Input: part model. Units: mm. Frame: model coordinates. A direction names the side the tool comes from. Give positions to 0.01 mm unless a question says otherwise; leave off trailing zeros. Order: outer loops, then holes, each group sorted by start corner. A loop starts at its lowest first (then second) coordinate and runs counter-clockwise, first axis right, second up.
```python
from build123d import *

# Parameters (mm, degrees)
PAD001_DEPTH    = 7.5
POCKET_DEPTH    = 17.001
CHAMFER002_SIZE = 0.5
CHAMFER003_SIZE = 0.5
FILLET002_R     = 0.5
FILLET003_R     = 0.5


with BuildPart() as part:
    # Sketch002 → Pad001 (new body, symmetric)
    with BuildSketch(Plane.XY):
        with BuildLine():
            ThreePointArc((-6.5, 3.741657), (0, -7.5), (6.5, 3.741657))
            ThreePointArc((8.233333, 4.739433), (6.867779, 5.107212), (6.5, 3.741657))
            ThreePointArc((7.690476, -5.577327), (9.486876, -0.49919), (8.233333, 4.739433))
            ThreePointArc((7.690476, -5.577327), (7.54881, -5.855807), (7.5, -6.164414))
            Line((7.5, -11.5), (7.5, -6.164414))
            Line((-7.5, -11.5), (7.5, -11.5))
            Line((-7.5, -6.164414), (-7.5, -11.5))
            ThreePointArc((-7.5, -6.164414), (-7.54881, -5.855807), (-7.690476, -5.577327))
            ThreePointArc((-8.233333, 4.739433), (-9.486876, -0.49919), (-7.690476, -5.577327))
            ThreePointArc((-6.5, 3.741657), (-6.867779, 5.107212), (-8.233333, 4.739433))
        make_face()
    extrude(amount=PAD001_DEPTH, both=True)

    # Sketch003 (on Face6 of Pad001) → Pocket (cut, through all)
    with BuildSketch(Plane.YZ.offset(7.5)):
        Polygon((-11.5, -3.237009), (-11.5, 3.237009), (-8.1, 5.2), (-8.1, -5.2), align=None)
    extrude(amount=-POCKET_DEPTH, mode=Mode.SUBTRACT)

    # Chamfer002
    chamfer002_edges = [part.edges().sort_by_distance(p)[0] for p in [
        (7.5, -11.5, 5.368505),
        (7.5, -9.8, 4.218505),
        (7.5, -8.1, 0),
        (7.5, -9.8, -4.218505),
        (7.5, -11.5, -5.368505),
    ]]
    chamfer(chamfer002_edges, length=CHAMFER002_SIZE)

    # Chamfer003
    chamfer003_edges = [part.edges().sort_by_distance(p)[0] for p in [
        (-7.5, -11.5, -5.368505),
        (-7.5, -9.8, -4.218505),
        (-7.5, -8.1, 0),
        (-7.5, -9.8, 4.218505),
        (-7.5, -11.5, 5.368505),
    ]]
    chamfer(chamfer003_edges, length=CHAMFER003_SIZE)

    # Fillet002
    fillet002_edges = [part.edges().sort_by_distance(p)[0] for p in [
        (6.867779, 5.107212, -7.5),
    ]]
    fillet(fillet002_edges, radius=FILLET002_R)

    # Fillet003
    fillet003_edges = [part.edges().sort_by_distance(p)[0] for p in [
        (6.867779, 5.107212, 7.5),
    ]]
    fillet(fillet003_edges, radius=FILLET003_R)


solid = part.part
```
1) Line query: probe 1 along X at (y, z) = (0, 2.25); probe 2 along X at (y, z) = (-1, 5); probe 3 along Y at (x, z) = (0, -1.5). Output: solid intervals per line, ascending.
2) Reachability of faces 5 (the face through (0, -8.1, 0)), 6 (the face through (-7.247, -9.577, -4.632)), 7 (the face through (-7.5, -7, 0)) from +Z, -Z, +X, -X, +Y, -Y: full face, straight path, thin tool, end or side. Return the list, or none.
3) First-contact query: P1, Ø5, axis at y = -7.5, z = -0.5, coming from the -X side; P2, Ø5.5, axis at y = -8, z = -1.5, coming from the +X side. Flat tips, straight axial feed; report the tip coordinate or a pass-through.
4) Pull-direction query (X, two-part tool) for faces 1 (the face through (9.483, -0.576, 0.098)), 2 (the face through (6.89, 5.12, 0.1)), 3 (the face through (0.1, -9.78, -4.23)), 4 (the face through (-0.22, -7.497, 0.098)); classes: pulls with the +X half, pulls with the -X half, needs draft (parallel to the pull), parting line crosses it, or undercut.
5) Cut plane B-B (z = -4.75). Return the cut outline in (x, y), then the cut area to 3 significant figures.
6) Cut plane C-C (z = 1.5). Return the cut outline in (x, y).
7) Cut plane A-A (x = 0). Return the cut outline in (y, z), then the cut area to 3 significant figures.
Geometry says:
1. probe 1: x = -9.5 to -7.5, 7.5 to 9.5
1. probe 2: x = -9.45 to -7.43, 7.43 to 9.45
1. probe 3: y = -8.1 to -7.5
2. face 5: +X, -X
2. face 6: -X
2. face 7: +Z, -Z, -X, -Y
3. P1: stops at x = -8.08
3. P2: stops at x = 7.92
4. face 1: pulls with the +X half
4. face 2: undercut
4. face 3: needs draft
4. face 4: undercut
5. outline: (-8.23, 4.74) arc R9.5 ccw to (-7.69, -5.58) arc R1 cw to (-7.5, -6.16) - (-7.5, -7.6) - (-7, -8.1) - (7, -8.1) - (7.5, -7.6) - (7.5, -6.16) arc R1 cw to (7.69, -5.58) arc R9.5 ccw to (8.23, 4.74) arc R1 ccw to (6.5, 3.74) arc R7.5 cw (long way) to (-6.5, 3.74) arc R1 ccw to start; (-7.5, -11) - (-7, -11.5) - (7, -11.5) - (7.5, -11) - (7.5, -9.88) - (7, -8.88) - (-7, -8.88) - (-7.5, -9.88) - close
5. area: 108 mm2
6. outline: (-8.23, 4.74) arc R9.5 ccw to (-7.69, -5.58) arc R1 cw to (-7.5, -6.16) - (-7.5, -7.6) - (-7, -8.1) - (7, -8.1) - (7.5, -7.6) - (7.5, -6.16) arc R1 cw to (7.69, -5.58) arc R9.5 ccw to (8.23, 4.74) arc R1 ccw to (6.5, 3.74) arc R7.5 cw (long way) to (-6.5, 3.74) arc R1 ccw to start
7. outline: (-11.5, -7.5) - (-8, -7.5) arc R0.5 ccw to (-7.5, -7) - (-7.5, 7) arc R0.5 ccw to (-8, 7.5) - (-11.5, 7.5) - (-11.5, 3.24) - (-8.1, 5.2) - (-8.1, -5.2) - (-11.5, -3.24) - close
7. area: 31.2 mm2
